from build123d import *

# Parameters (mm, degrees)
SKETCH1_W               = 139.7
SKETCH1_H               = 12.7
BOSS_EXTRUDE1_DEPTH     = 146.05
SKETCH2_W               = 12.7
SKETCH2_H               = 6.35
BOSS_EXTRUDE2_DEPTH     = 19.05
CUT_EXTRUDE4_REACH      = 213.847
SKETCH6_R               = 3.175
FILLET1_R               = 2.54
SKETCH3_R               = 16.764
CUT_EXTRUDE5_DEPTH      = 10.16
SKETCH7_R               = 11.4554
CUT_EXTRUDE6_DEPTH      = 216.952287786
BOSS_EXTRUDE3_DEPTH     = 12.7
MIRROR3_COPY_1_REACH    = 213.847
MIRROR3_COPY_1_SKETCH_R = 3.175
SKETCH10_R              = 3.3782
CUT_EXTRUDE8_DEPTH      = 218.203418481
SKETCH11_R              = 4.826
CUT_EXTRUDE9_DEPTH      = 6.35
SKETCH12_R              = 11.4554
CUT_EXTRUDE10_DEPTH     = 217.086683995


with BuildPart() as part:
    # Sketch1 → Boss-Extrude1 (new body)
    with BuildSketch(Plane(origin=(0, 0, 0), x_dir=(1, 0, 0), z_dir=(0, 1, 0))):
        with Locations((69.85, 6.35)):
            Rectangle(SKETCH1_W, SKETCH1_H)
    extrude(amount=BOSS_EXTRUDE1_DEPTH)

    # Sketch2 → Boss-Extrude2 (add)
    with BuildSketch(Plane.ZY):
        with Locations((-6.35, 3.175)):
            Rectangle(SKETCH2_W, SKETCH2_H)
    boss_extrude2 = extrude(amount=BOSS_EXTRUDE2_DEPTH)

    # Mirror1: Boss-Extrude2 across plane
    add(boss_extrude2.mirror(Plane.ZY.offset(-69.85)))

    # Sketch6 → Cut-Extrude4 (cut, up to next)
    with BuildSketch(Plane(origin=(0, 6.35, 0), x_dir=(1, 0, 0), z_dir=(0, 1, 0)), mode=Mode.PRIVATE) as cut_extrude4_sk1:
        with Locations(Location((-9.906, 6.35, 0), (0, 0, 270))):
            Circle(SKETCH6_R)
    cut_extrude4_tool1 = extrude(cut_extrude4_sk1.sketch, amount=-CUT_EXTRUDE4_REACH, mode=Mode.PRIVATE) & part.part
    cut_extrude4 = cut_extrude4_tool1.solids().sort_by_distance((-9.906, 6.35, -6.35))[0]
    add(cut_extrude4, mode=Mode.SUBTRACT)

    # Mirror2: Cut-Extrude4 across plane
    add(cut_extrude4.mirror(Plane.ZY.offset(-69.85)), mode=Mode.SUBTRACT)

    # Fillet1
    fillet1_edges = [part.edges().sort_by_distance(p)[0] for p in [
        (139.7, 146.05, -6.35),
        (-19.05, 6.35, -6.35),
        (158.75, 6.35, -6.35),
        (0, 146.05, -6.35),
    ]]
    fillet(fillet1_edges, radius=FILLET1_R)

    # Sketch3 → Cut-Extrude5 (cut)
    with BuildSketch(Plane.XY):
        with Locations((69.85, 76.2)):
            Circle(SKETCH3_R)
    extrude(amount=-CUT_EXTRUDE5_DEPTH, mode=Mode.SUBTRACT)

    # Sketch7 → Cut-Extrude6 (cut, through all)
    with BuildSketch(Plane.XY.offset(-10.16)):
        with Locations((69.85, 76.2)):
            Circle(SKETCH7_R)
    extrude(amount=-CUT_EXTRUDE6_DEPTH, mode=Mode.SUBTRACT)

    # Sketch8 → Boss-Extrude3 (add)
    with BuildSketch(Plane(origin=(0, 0, -12.7), x_dir=(-1, 0, 0), z_dir=(0, 0, -1))):
        with BuildLine():
            Line((-137.16, 146.05), (-2.54, 146.05))
            ThreePointArc((-2.54, 146.05), (-0.743948776, 145.306051224), (0, 143.51))
            Line((0, 143.51), (0, 6.35))
            Line((0, 6.35), (16.51, 6.35))
            ThreePointArc((16.51, 6.35), (18.306051224, 5.606051224), (19.05, 3.81))
            Line((19.05, 3.81), (19.05, 0))
            Line((19.05, 0), (-158.75, 0))
            Line((-158.75, 0), (-158.75, 3.81))
            ThreePointArc((-158.75, 3.81), (-158.006051224, 5.606051224), (-156.21, 6.35))
            Line((-156.21, 6.35), (-139.7, 6.35))
            Line((-139.7, 6.35), (-139.7, 143.51))
            ThreePointArc((-139.7, 143.51), (-138.956051224, 145.306051224), (-137.16, 146.05))
        make_face()
    extrude(amount=BOSS_EXTRUDE3_DEPTH)

    # Mirror3: Cut-Extrude4 across plane
    add(cut_extrude4.mirror(Plane(origin=(0, 0, -12.7), x_dir=(1, 0, 0), z_dir=(0, 0, -1))), mode=Mode.SUBTRACT)

    # Mirror3 copy 1 sketch → Mirror3 copy 1 (cut, up to next)
    with BuildSketch(Plane(origin=(139.7, 6.35, -25.4), x_dir=(-1, 0, 0), z_dir=(0, 1, 0)), mode=Mode.PRIVATE) as mirror3_copy_1_sk1:
        with Locations(Location((-9.906, 6.35, 0), (0, 0, 270))):
            Circle(MIRROR3_COPY_1_SKETCH_R)
    mirror3_copy_1_tool1 = extrude(mirror3_copy_1_sk1.sketch, amount=-MIRROR3_COPY_1_REACH, mode=Mode.PRIVATE) & part.part
    add(mirror3_copy_1_tool1.solids().sort_by_distance((149.606, 6.35, -19.05))[0], mode=Mode.SUBTRACT)

    # Sketch10 → Cut-Extrude8 (cut, through all)
    with BuildSketch(Plane.XY):
        with Locations((11.43, 76.2)):
            Circle(SKETCH10_R)
        with Locations((69.85, 134.62)):
            Circle(SKETCH10_R)
        with Locations((128.27, 76.2)):
            Circle(SKETCH10_R)
        with Locations((69.85, 17.78)):
            Circle(SKETCH10_R)
    extrude(amount=-CUT_EXTRUDE8_DEPTH, mode=Mode.SUBTRACT)

    # Sketch11 → Cut-Extrude9 (cut)
    with BuildSketch(Plane.XY):
        with Locations((11.43, 76.2)):
            Circle(SKETCH11_R)
        with Locations((69.85, 134.62)):
            Circle(SKETCH11_R)
        with Locations((128.27, 76.2)):
            Circle(SKETCH11_R)
        with Locations((69.85, 17.78)):
            Circle(SKETCH11_R)
    extrude(amount=-CUT_EXTRUDE9_DEPTH, mode=Mode.SUBTRACT)

    # Sketch12 → Cut-Extrude10 (cut, through all)
    with BuildSketch(Plane.XY.offset(-12.7)):
        with Locations((69.85, 76.2)):
            Circle(SKETCH12_R)
    extrude(amount=-CUT_EXTRUDE10_DEPTH, mode=Mode.SUBTRACT)


solid = part.part
Check sheet for the modelled part. Datum: model origin and axes. Units: mm. A direction names the side the tool comes from. Round coordinates to 2 decimals unless told otherwise and drop trailing zeros. Order: outer loops, then holes, each group sorted by start corner. A loop starts at its lowest first (then second) coordinate and runs counter-clockwise, first axis right, second up.
(1) Draft check along Z on faces 6 (the flat face through (-8, 6.35, -13)), 7 (the flat face through (69, 56, 0)), 8 (the cylindrical face through (-7.23, 3.22, -4.64)). Enter one of: pulls with the +Z half, pulls with the -Z half, needs draft (parallel to the pull), parting line crosses it, or undercut.
(2) Cross-section at A-A, the plane y = 134.62. Enter the section's corners in (x, z).
(3) Scan lines: probe 1 along Y at (x, z) = (69.85, -19.25); probe 2 along X at (y, z) = (2, -19.05); probe 3 along X at (y, z) = (4.25, -19.05). Record each from-to range of solid material in increasing order.
(4) Cross-section at C-C, the plane x = 69.85. Enter the section's corners in (y, z).
(5) Cross-section at B-B, the plane y = 76.2. Enter the section's corners in (x, z), and give its area (3 significant figures).
(6) Access from +Z, -Z, +X, -X, +Y, -Y to the whole of each face (thin tool, end or side, straight path). Record for faces 1 (the flat face through (69, 90, -25.4)), 2 (the flat face through (8, 75, -6.35)), 3 (the cylindrical face through (12.989, 73.203, -15.742)), 4 (the flat face through (148, 6.35, -13)), 5 (the flat face through (0, 76, -13)).
(7) Go/stop test with flat-tipped pins: P1, Ø8, axis at x = 69.85, y = 134.62, coming from the +Z side; P2, Ø2, axis at y = 106.5, z = -21.5, coming from the +X side; P3, Ø10, axis at x = -9.906, z = -19.05, coming from the +Y side; P4, Ø5.5, axis at x = 149.606, z = -19.05, coming from the -Y side. Record where each tip stops, or that it passes through.
(8) Cross-section at D-D, the plane y = 117. Enter the section's corners in (x, z), and give its area (3 significant figures).
Check sheet entries:
1. face 6: needs draft
1. face 7: pulls with the +Z half
1. face 8: undercut
2. outline: (0, -25.4) - (66.47, -25.4) - (66.47, -6.35) - (65.02, -6.35) - (65.02, 0) - (0, 0) - close; (73.23, -25.4) - (139.7, -25.4) - (139.7, 0) - (74.68, 0) - (74.68, -6.35) - (73.23, -6.35) - close
3. probe 1: y = 0 to 14.4, 21.16 to 64.74, 87.66 to 131.24, 138 to 146.05
3. probe 2: x = -19.05 to -13.08, -6.73 to 146.43, 152.78 to 158.75
3. probe 3: x = -19.01 to -13.08, -6.73 to 146.43, 152.78 to 158.71
4. outline: (0, -25.4) - (14.4, -25.4) - (14.4, -6.35) - (12.95, -6.35) - (12.95, 0) - (0, 0) - close; (21.16, -25.4) - (64.74, -25.4) - (64.74, -10.16) - (59.44, -10.16) - (59.44, 0) - (22.61, 0) - (22.61, -6.35) - (21.16, -6.35) - close; (87.66, -25.4) - (131.24, -25.4) - (131.24, -6.35) - (129.79, -6.35) - (129.79, 0) - (92.96, 0) - (92.96, -10.16) - (87.66, -10.16) - close; (138, -25.4) - (146.05, -25.4) - (146.05, 0) - (139.45, 0) - (139.45, -6.35) - (138, -6.35) - close
5. outline: (0, -25.4) - (8.05, -25.4) - (8.05, -6.35) - (6.6, -6.35) - (6.6, 0) - (0, 0) - close; (14.81, -25.4) - (58.39, -25.4) - (58.39, -10.16) - (53.09, -10.16) - (53.09, 0) - (16.26, 0) - (16.26, -6.35) - (14.81, -6.35) - close; (81.31, -25.4) - (124.89, -25.4) - (124.89, -6.35) - (123.44, -6.35) - (123.44, 0) - (86.61, 0) - (86.61, -10.16) - (81.31, -10.16) - close; (131.65, -25.4) - (139.7, -25.4) - (139.7, 0) - (133.1, 0) - (133.1, -6.35) - (131.65, -6.35) - close
5. area: 2,480 mm2
6. face 1: -Z, +X, -X, +Y, -Y
6. face 2: +Z
6. face 3: +Z, -Z
6. face 4: +Z, -Z, +X, +Y
6. face 5: +Z, -Z, -X, +Y
7. P1: stops at z = -6.35
7. P2: stops at x = 139.7
7. P3: stops at y = 6.35
7. P4: passes through
8. outline: (0, -25.4) - (139.7, -25.4) - (139.7, 0) - (0, 0) - close
8. area: 3,550 mm2
